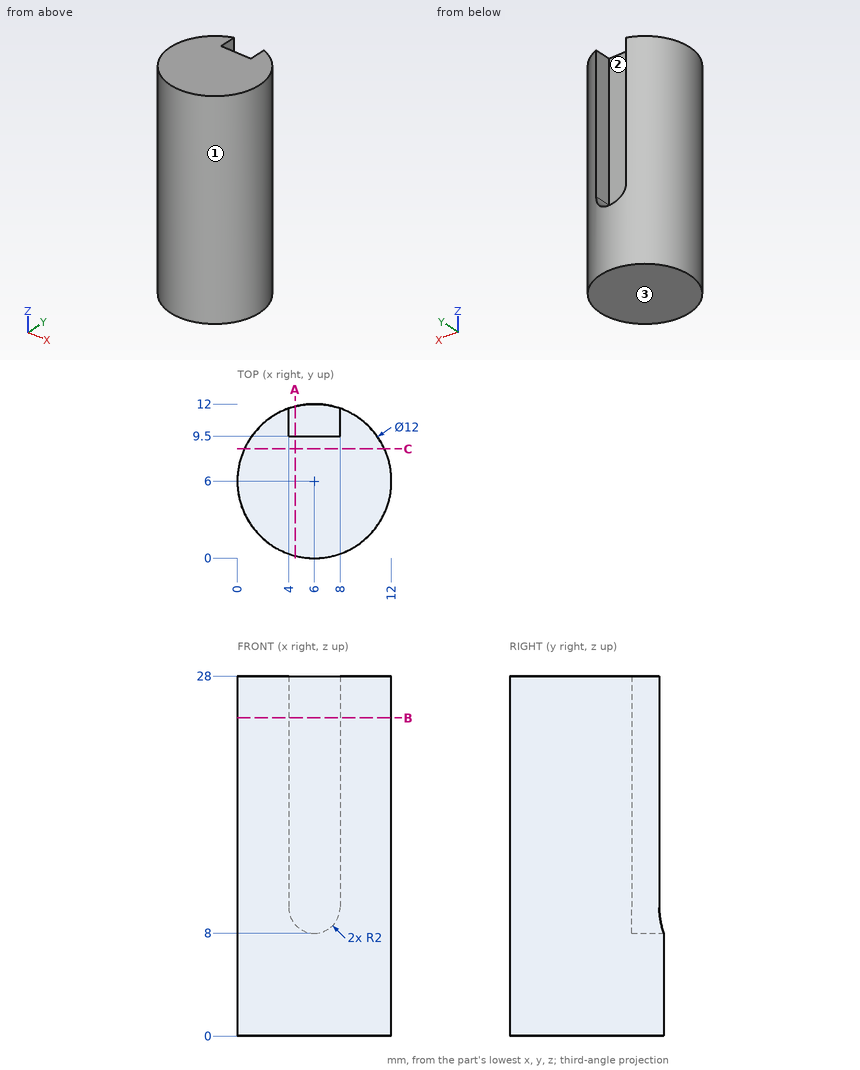
Design review of the part shown in the three views and the two pictorial views. Dimensions are in mm from the part's minimum x, y and z. Give positions to 0.01 mm unless a question says otherwise; leave off trailing zeros. Loops run counter-clockwise (first coordinate to the right, second up) from the corner with the lowest first, then second, coordinate; pieces in that order, holes last. Notation, with made-up numbers: (-1, 10) - (44, 10) arc R23 ccw to (44, 41) - close; hole circle Ø4 at (-29.75, -37). An arc over 180 degrees is marked (long way). Use CSV: the item, a comma, the result in double quotes. Start each with the question number.
1. Wall thickness on L1, parallel to Y at x = 5.75, z = 3.25 (3 decimals); L2, parallel to X at y = 9.75, z = 19.75; L3, parallel to X at y = 10.25, z = 8.75 (1 decimal): over which ranges is each line inside the solid? List them lowest first.
2. Insertion check: P1, Ø2.5, axis at y = 11, z = 20, coming from the -X side; P2, Ø2.5, axis at y = 10, z = 22.5, coming from the +X side; P3, Ø3, axis at y = 8, z = 15, coming from the +X side. Each pin has a flat end and moves straight along its axis. Give the tip position at first contact, or say it passes through.
3. Add section B-B (z = 24.75). State the section outline as (x, y) points.
4. Add section A-A (x = 4.5). State the section outline as (y, z) points.
5. Draft analysis for pull direction X (two halves, no side actions). For the marked faces 1, 2 and 3, state which applies: released by +X, released by -X, zero draft, split by the parting line, or undercut.
6. Add section C-C (y = 8.5). State the section outline as (x, z) points.
Results found:
1,L1,"y = 0.005 to 11.995"
1,L2,"x = 1.32 to 4, 8 to 10.68"
1,L3,"x = 1.8 to 4.4, 7.6 to 10.2"
2,P1,"stops at x = 1.32"
2,P2,"stops at x = 11.33"
2,P3,"stops at x = 11.98"
3,outline,"(4, 9.5) - (4, 11.66) arc R6 ccw (long way) to (8, 11.66) - (8, 9.5) - close"
4,outline,"(0.19, 0) - (11.81, 0) - (11.81, 8.68) - (9.5, 8.68) - (9.5, 28) - (0.19, 28) - close"
5,face 1,"split by the parting line"
5,face 2,"undercut"
5,face 3,"zero draft"
6,outline,"(0.55, 0) - (11.45, 0) - (11.45, 28) - (0.55, 28) - close"
